from build123d import *

# Parameters (mm, degrees)
SKETCH1_R           = 5
BOSS_EXTRUDE1_DEPTH = 3
SKETCH3_R           = 3.8
CUT_EXTRUDE1_DEPTH  = 1.8
SKETCH4_R           = 2
BOSS_EXTRUDE2_DEPTH = 4
SKETCH5_R           = 1
CUT_EXTRUDE2_DEPTH  = 4
SKETCH6_W           = 4
SKETCH6_H           = 4
CUT_EXTRUDE3_DEPTH  = 1.2
CHAMFER1_SIZE       = 1


with BuildPart() as part:
    # Sketch1 → Boss-Extrude1 (new body)
    with BuildSketch(Plane(origin=(0, 0, 0), x_dir=(1, 0, 0), z_dir=(0, 1, 0))):
        Circle(SKETCH1_R)
    extrude(amount=BOSS_EXTRUDE1_DEPTH)

    # Sketch3 → Cut-Extrude1 (cut)
    with BuildSketch(Plane(origin=(0, 3, 0), x_dir=(1, 0, 0), z_dir=(0, 1, 0))):
        Circle(SKETCH3_R)
    extrude(amount=-CUT_EXTRUDE1_DEPTH, mode=Mode.SUBTRACT)

    # Sketch4 → Boss-Extrude2 (add)
    with BuildSketch(Plane(origin=(0, 1.2, 0), x_dir=(1, 0, 0), z_dir=(0, 1, 0))):
        Circle(SKETCH4_R)
    extrude(amount=BOSS_EXTRUDE2_DEPTH)

    # Sketch5 → Cut-Extrude2 (cut)
    with BuildSketch(Plane(origin=(0, 5.2, 0), x_dir=(1, 0, 0), z_dir=(0, 1, 0))):
        Circle(SKETCH5_R)
    extrude(amount=-CUT_EXTRUDE2_DEPTH, mode=Mode.SUBTRACT)

    # Sketch6 → Cut-Extrude3 (cut)
    with BuildSketch(Plane(origin=(0, 3, 0), x_dir=(1, 0, 0), z_dir=(0, 1, 0))):
        with Locations((4, 0)):
            Rectangle(SKETCH6_W, SKETCH6_H)
    extrude(amount=-CUT_EXTRUDE3_DEPTH, mode=Mode.SUBTRACT)

    # Chamfer1
    chamfer1_edges = [part.edges().sort_by_distance(p)[0] for p in [
        (-5, 0, 0),
    ]]
    chamfer(chamfer1_edges, length=CHAMFER1_SIZE)


solid = part.part
Input: part model. Units: mm. Frame: model coordinates. A direction names the side the tool comes from. Coordinates: 2 decimals unless noted, no trailing zeros. Loops run counter-clockwise (first coordinate to the right, second up) from the corner with the lowest first, then second, coordinate; pieces in that order, holes last. Notation, with made-up numbers: (88.5, 51) -> (112.5, 51) arc R16 ccw to (112.5, 60) -> close; hole circle Ø1 at (53, -34). An arc over 180 degrees is marked (long way). Write each question's results on one line, items separated by ' | '. Start each with the question number.
Q1. Section C-C, the plane y = 1.55. Return the cut outline in (x, z), plus the area to 3 significant figures.
Q2. Section B-B, the plane x = 0. Return the cut outline in (y, z), plus the area to 3 significant figures.
Q3. Ray query, line 1 (Z direction, x = 0, y = 1.65); line 2 (X direction, y = 2.6, z = 0). Return the intervals inside material, ascending. Write a range as from..to.
Q4. Section A-A, the plane y = 2.1. Return the cut outline in (x, z).
Q5. Reachability of faces 4 (the flat face through (4, 2, 2)), 5 (the cylindrical face through (-3.796, 2.113, -0.167)), 6 (the flat face through (0, 0, 0)) from +Z, -Z, +X, -X, +Y, -Y: full face, straight path, thin tool, end or side. Return the list, or none.
Q6. Section D-D, the plane z = 0. Return the cut outline in (x, y).
Q7. Pull-direction query (Z, two-part tool) for faces 1 (the cylindrical face through (0, 3, 1)), 2 (the cylindrical face through (-5, 2, 0)), 3 (the flat face through (-4, 3, 1)); classes: released by +Z, released by -Z, zero draft, split by the parting line, or undercut.
Q8. Pin query (flat end, axial travel): pin 1 (3 mm diameter, centred on x = -3.5, z = 1, fed in from +Y); pin 2 (1 mm diameter, centred on x = 3.5, y = 2.5, fed in from +Z); pin 3 (1.3 mm diameter, centred on x = 4, y = 2.5, fed in from -Z). Return the tip coordinate at first contact, or that it passes through.
Found:
1) outline: circle Ø10 at (0, 0); circle Ø4 at (0, 0); hole circle Ø7.6 at (0, 0); hole circle Ø2 at (0, 0) | area: 42.6 mm2
2) outline: (0, -4) -> (1, -5) -> (3, -5) -> (3, -3.8) -> (1.2, -3.8) -> (1.2, -2) -> (5.2, -2) -> (5.2, -1) -> (1.2, -1) -> (1.2, 1) -> (5.2, 1) -> (5.2, 2) -> (1.2, 2) -> (1.2, 3.8) -> (3, 3.8) -> (3, 5) -> (1, 5) -> (0, 4) -> close | area: 23.3 mm2
3) line 1: -5..-3.8, -2..-1, 1..2, 3.8..5 | line 2: -5..-3.8, -2..-1, 1..2
4) outline: circle Ø4 at (0, 0); (3.23, -2) arc R3.8 cw (long way) to (3.23, 2) -> (4.58, 2) arc R5 ccw (long way) to (4.58, -2) -> close; hole circle Ø2 at (0, 0)
5) face 4: +X, +Y | face 5: +Y | face 6: +Z, -Z, +X, -X, -Y
6) outline: (-5, 1) -> (-4, 0) -> (4, 0) -> (5, 1) -> (5, 1.8) -> (3.8, 1.8) -> (3.8, 1.2) -> (2, 1.2) -> (2, 5.2) -> (1, 5.2) -> (1, 1.2) -> (-1, 1.2) -> (-1, 5.2) -> (-2, 5.2) -> (-2, 1.2) -> (-3.8, 1.2) -> (-3.8, 3) -> (-5, 3) -> close
7) face 1: undercut | face 2: split by the parting line | face 3: zero draft
8) pin 1: y = 3 | pin 2: z = 4 | pin 3: z = -3.71
